Read the model definition and answer for the solid it produces. Units are mm, in the model's axes. A direction names the side the tool comes from. Coordinates: 2 decimals unless noted, no trailing zeros. Loops run counter-clockwise (first coordinate to the right, second up) from the corner with the lowest first, then second, coordinate; pieces in that order, holes last. Notation, with made-up numbers: (-39, 1) - (-1, 1) arc R21 cw to (-1, 8) - close; hole circle Ø1 at (79, -5). An arc over 180 degrees is marked (long way). Use CSV: the item, a comma, the result in double quotes.
```python
from build123d import *

# Parameters (mm, degrees)
F0_W     = 914.4
F0_H     = 76.2
F1_DEPTH = 177.8
F3_DEPTH = 2133.6
F4_W     = 25.4
F4_H     = 12.7
F5_DEPTH = 2438.4


with BuildPart() as f1:
    # F0 (on Top) → F1 (new body)
    with BuildSketch(Plane.XY):
        with Locations((325.290451, 32.179302)):
            Rectangle(F0_W, F0_H)
    extrude(amount=F1_DEPTH)

    # F2 (on face) → F3 (cut)
    with BuildSketch(Plane.YZ.offset(782.490451)):
        Polygon((32.179302, 88.9), (-5.920698, 152.4), (-5.920698, 0), (32.179302, 0), align=None)
    extrude(amount=-F3_DEPTH, mode=Mode.SUBTRACT)

    # F4 (on face) → F5 (cut)
    with BuildSketch(Plane.YZ.offset(782.490451)):
        with Locations((6.779302, 171.45)):
            Rectangle(F4_W, F4_H)
    extrude(amount=-F5_DEPTH, mode=Mode.SUBTRACT)


solid = f1.part
```
Q1. The part is cut by section C-C on y = 9.5. Determine the outline of the cut face in (x, z), and give its area (3 significant figures).
Reported:
outline,"(-131.91, 126.7) - (782.49, 126.7) - (782.49, 165.1) - (-131.91, 165.1) - close"
area,"35,100 mm²"
Q2. The part is cut by section B-B on z = 16.5. Determine the outline of the cut face in (x, y), and give its area (3 significant figures).
Reported:
outline,"(-131.91, 32.18) - (782.49, 32.18) - (782.49, 70.28) - (-131.91, 70.28) - close"
area,"34,800 mm²"
Q3. Given P1, Ø6.5, axis at x = 235, z = 169, coming from the -Y side; P2, Ø2, axis at x = 179.5, y = 37.5, coming from the -Z side; P3, Ø12.5, axis at x = 435.5, y = 5, coming from the +Z side; P4, Ø5, axis at x = 73, y = 17.5, coming from the -Z side, each flat-ended and moving along its own axis, determine where each tip first touches the part or whether it passes through.
Reported:
P1,"stops at y = 19.48"
P2,"stops at z = 0"
P3,"stops at z = 165.1"
P4,"stops at z = 109.2"
Q4. A tool of negligible diameter and unlimited length cuts with its end or side. For faces 1 (the face through (332, 7, 165.1)), 2 (the face through (319, 45, 177.8)), 3 (the face through (332, 32.179, 44)), from which of +Z, -Z, +X, -X, +Y, -Y can it reach the whole face along a straight path? Write none if from no direction.
Reported:
face 1,"+Z, +X, -X, -Y"
face 2,"+Z, +X, -X, +Y, -Y"
face 3,"-Z, +X, -X, -Y"
Q5. The part is cut by section A-A on x = 683. Determine the outline of the cut face in (y, z).
Reported:
outline,"(-5.92, 152.4) - (32.18, 88.9) - (32.18, 0) - (70.28, 0) - (70.28, 177.8) - (19.48, 177.8) - (19.48, 165.1) - (-5.92, 165.1) - close"
Q6. Find the intervals of material crossed by probe 1 along Y at (x, z) = (508.5, 76); probe 2 along Z at (x, y) = (-46, -0.5); probe 3 along Z at (x, y) = (477.5, 24.5), in increasing order. Write a range as [from, to].
Reported:
probe 1,"y = [32.18, 70.28]"
probe 2,"z = [143.37, 165.1]"
probe 3,"z = [101.7, 177.8]"
